Geometry: final body of the model. Coordinates: model frame, mm. Face numbers are marked on the shaded views. A direction names the side the tool comes from. Coordinates: 2 decimals unless noted, no trailing zeros. Write each loop counter-clockwise with the first axis right and the second up, starting at its lowest first coordinate (ties: lowest second). Pieces come first, ordered by that corner, then holes.
Autodesk Inventor part; units mm, degrees
ref_plane "YZ Plane" through (0, 0, 0) normal (1, 0, 0) x (0, 1, 0)
ref_plane "XZ Plane" through (0, 0, 0) normal (0, 1, 0) x (-1, 0, 0)
ref_plane "XY Plane" through (0, 0, 0) normal (0, 0, 1) x (1, 0, 0)
sketch "Sketch1" plane through (0, 0, 0) normal (0, 0, 1) x (1, 0, 0)
  line L0 (-100.0125, -209.55) -> (100.0125, -209.55)
  line L1 (100.0125, -209.55) -> (100.0125, 209.55)
  line L2 (100.0125, 209.55) -> (-100.0125, 209.55)
  line L3 (-100.0125, 209.55) -> (-100.0125, -209.55)
  circle A0 centre (69.85, 203.2) radius 3.175
  line L4 (66.675, 209.55) -> (73.025, 209.55)
  line L5 (73.025, 209.55) -> (73.025, 203.2)
  line L6 (73.025, 203.2) -> (66.675, 203.2)
  line L7 (66.675, 203.2) -> (66.675, 209.55)
  line L8 (0, 209.55) -> (0, -209.55)
  line L9 (100.0125, 0) -> (-100.0125, 0)
  circle A1 centre (-69.85, 203.2) radius 3.175
  line L10 (-66.675, 209.55) -> (-73.025, 209.55)
  line L11 (-73.025, 209.55) -> (-73.025, 203.2)
  line L12 (-73.025, 203.2) -> (-66.675, 203.2)
  line L13 (-66.675, 203.2) -> (-66.675, 209.55)
  circle A2 centre (69.85, -203.2) radius 3.175
  line L14 (66.675, -209.55) -> (73.025, -209.55)
  line L15 (73.025, -209.55) -> (73.025, -203.2)
  line L16 (73.025, -203.2) -> (66.675, -203.2)
  line L17 (66.675, -203.2) -> (66.675, -209.55)
  circle A3 centre (-69.85, -203.2) radius 3.175
  line L18 (-66.675, -209.55) -> (-73.025, -209.55)
  line L19 (-73.025, -209.55) -> (-73.025, -203.2)
  line L20 (-73.025, -203.2) -> (-66.675, -203.2)
  line L21 (-66.675, -203.2) -> (-66.675, -209.55)
  point P0 (0, 0)
  point P1 (0, 0)
  dimension "d0" = 419.1
  dimension "d1" = 200.025
  dimension "d2" = 6.35
  dimension "d3" = 6.35
  dimension "d4" = 30.1625
extrude "Extrusion1" add sketch "Sketch1" along normal blind 1.5875 contours L3 L9 L8 L0 L21 A3 L19 | L3 L2 L11 A1 L13 L8 L9 | L9 L1 L0 L15 A2 L17 L8 | L8 L2 L7 A0 L5 L1 L9
sketch "Sketch2" plane through (0, 0, 1.5875) normal (0, 0, 1) x (1, 0, 0)
  line L0 (100.0125, 209.55) -> (100.0125, -209.55)
  line L1 (-100.0125, -209.55) -> (-100.0125, 209.55)
  line L2 (-100.0125, 190.5) -> (100.0125, 190.5)
  line L3 (100.0125, 190.5) -> (100.0125, -190.5)
  line L4 (100.0125, -190.5) -> (-100.0125, -190.5)
  line L5 (-100.0125, -190.5) -> (-100.0125, 190.5)
  point P0 (0, 0)
  point P1 (-100.0125, 0)
  dimension "d7" = 381
extrude "Extrusion2" add sketch "Sketch2" along normal blind 77.7875
sketch "Sketch3" plane through (-100.0125, -190.5, 1.5875) normal (0, -1, 0) x (1, 0, 0)
  line L0 (0, 0) -> (0, 77.7875)
  circle A0 centre (19.05, 42.8625) radius 9.525
  line L1 (0, -1.5875) -> (26.9875, -1.5875)
  point P0 (100.0125, -1.5875)
  dimension "d10" = 19.05
  dimension "d11" = 44.45
  dimension "d12" = 19.05
extrude "Extrusion3" add sketch "Sketch3" along normal blind 33.3375
mirror "Mirror1" about plane through (0, 0, 0) normal (1, 0, 0) of "Extrusion3"
properties part number "2kW inverter"
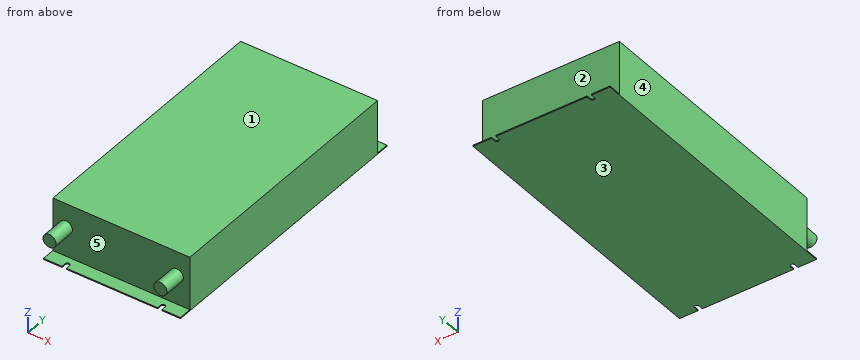
Item 1: Section C-C, the plane z = 15. Output: boundary loops of the cut face in (x, y).
Derived:
outline: (-100.01, -190.5) - (100.01, -190.5) - (100.01, 190.5) - (-100.01, 190.5) - close
Item 2: Material intervals for probe 1 along Y at (x, z) = (-91, 65); probe 2 along Y at (x, z) = (-83.5, 51), sorted ascending.
Derived:
probe 1: y = -190.5 to 190.5
probe 2: y = -223.84 to 190.5
Item 3: Pull-direction query (X, two-part tool) for the marked faces 3, 4 and 5; classes: released by +X, released by -X, zero draft, split by the parting line, or undercut.
Derived:
face 3: zero draft
face 4: released by -X
face 5: undercut
Item 4: Pin query (flat end, axial travel): pin 1 (1.7 mm diameter, centred on x = 29, z = 0.5, fed in from -Y); pin 2 (21 mm diameter, centred on x = -34.5, y = -203.5, fed in from +Z); pin 3 (2 mm diameter, centred on x = -67, z = 30, fed in from -Y). Return the tip coordinate at first contact, or that it passes through.
Derived:
pin 1: stops at y = -209.55
pin 2: stops at z = 1.59
pin 3: stops at y = -190.5
Item 5: Set-up query: the marked faces 1 and 2. Return all of +Z, -Z, +X, -X, +Y, -Y with unobstructed straight access to the full face (end or side cutting, diameter ignored); none if empty.
Derived:
face 1: +Z, +X, -X, +Y, -Y
face 2: +Z, +X, -X, +Y
Item 6: Section A-A, the plane z = 44.45. Output: boundary loops of the cut face in (x, y), plus the area to 3 significant figures.
Derived:
outline: (-100.01, -190.5) - (-90.49, -190.5) - (-90.49, -223.84) - (-71.44, -223.84) - (-71.44, -190.5) - (71.44, -190.5) - (71.44, -223.84) - (90.49, -223.84) - (90.49, -190.5) - (100.01, -190.5) - (100.01, 190.5) - (-100.01, 190.5) - close
area: 77,500 mm2
